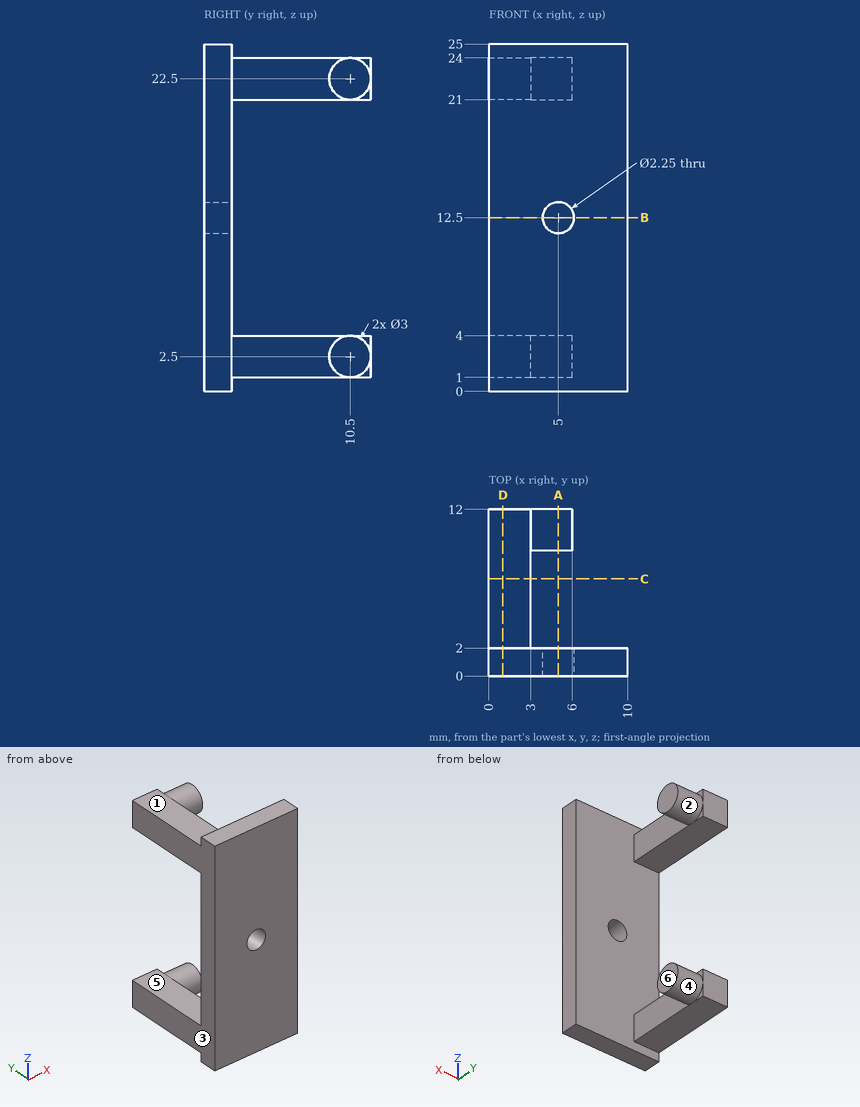
The drawing under review shows one solid part. Ordinate dimensions are in mm from its lowest x, y, z. A direction names the side the tool comes from. Round coordinates to 2 decimals unless told otherwise and drop trailing zeros. Write each loop counter-clockwise with the first axis right and the second up, starting at its lowest first coordinate (ties: lowest second). Pieces come first, ordered by that corner, then holes. Notation, with made-up numbers: M -6.75,41.25 L 3.25,41.25 A20 ccw 3.25,54.25 Z; hole C -31,75 d7. An arc over 180 degrees is marked long. One line per item, written item: value. Start each with the question number.
(1) Wall thickness on line 1 (Z direction, x = 5, y = 1.1) (3 decimals); line 2 (X direction, y = 0.75, z = 12.5) (3 decimals); line 3 (Y direction, x = 8.5, z = 7.5): over which ranges is each line inside the solid? List them lowest first.
(2) We need section C-C (y = 7). Give the boundary of the cut face in (x, z), and give its area (3 significant figures).
(3) Machinability: for the marked faces 4, 5 and 6, which of the approach directions +Z, -Z, +X, -X, +Y, -Y give a long, thin tool a straight path to every point of the face, cutting with its end or side? Answer none if there is none.
(4) Insertion check: pin 1 (1.5 mm diameter, centred on y = 10.5, z = 3, fed in from +X); pin 2 (3.5 mm diameter, centred on x = 1, y = 8.5, fed in from +Z); pin 3 (1.5 mm diameter, centred on x = 1, y = 7, fed in from -Z). Each pin has a flat end and moves straight along its axis. Give the tip position at first contact, or say it passes through.
(5) We need section B-B (z = 12.5). Give the boundary of the cut face in (x, y) (3 decimals).
(6) We need section D-D (x = 1). Give the boundary of the cut face in (y, z).
(7) We need section A-A (x = 5). Give the boundary of the cut face in (y, z) (3 decimals), and give its area (3 significant figures).
(8) The part is to be moulded in two halves that separate along Z. For the marked faces 1, 2 and 3, say which applies: released by +Z, released by -Z, zero draft, split by the parting line, or undercut.
Result:
1. line 1: 0 to 11.375, 13.625 to 25
1. line 2: 0 to 3.875, 6.125 to 10
1. line 3: 0 to 2
2. outline: M 0,1 L 3,1 L 3,4 L 0,4 Z; M 0,21 L 3,21 L 3,24 L 0,24 Z
2. area: 18.0 mm²
3. face 4: +X
3. face 5: +X, -X, +Y
3. face 6: +Z, -Z, +X, +Y
4. pin 1: x = 6
4. pin 2: z = 24
4. pin 3: z = 1
5. outline: M 0,0 L 3.875,0 L 3.875,2 L 0,2 Z; M 6.125,0 L 10,0 L 10,2 L 6.125,2 Z
6. outline: M 0,0 L 2,0 L 2,1 L 12,1 L 12,4 L 2,4 L 2,21 L 12,21 L 12,24 L 2,24 L 2,25 L 0,25 Z
7. outline: M 0,0 L 2,0 L 2,11.375 L 0,11.375 Z; M 0,13.625 L 2,13.625 L 2,25 L 0,25 Z; C 10.5,2.5 d3; C 10.5,22.5 d3
7. area: 59.6 mm²
8. face 1: released by +Z
8. face 2: undercut
8. face 3: zero draft
